Could you check a few things on this model? Use its own coordinates, in mm. A direction names the side the tool comes from. Coordinates: 2 decimals unless noted, no trailing zeros. One line per question, with ' | ' between items. Start each with the question number.
(1) I'm going to push flat-ended pins straight in: pin 1 Ø2.5 at (x, y) = (-150.5, 0.5) entering from -Z; pin 2 Ø10 at (x, z) = (-102, 42.5) entering from +Y; pin 3 Ø3 at (y, z) = (-116, -54) entering from +X. Where does each tip first touch, or does it pass through?
(2) If we mould it in two halves opening along X, with no side actions, what happens to faces 1 (the face through (-24, -8, 132.5)), 2 (the face through (-4, 1, 167.5)), 3 (the face through (-3.78, -130.33, -2.72))? For each: pulls with the +X half, pulls with the -X half, needs draft (parallel to the pull), parting line crosses it, or undercut.
(3) If I drill on line 1 along X through (y, z) = (24, 73.5); line 2 along X through (y, z) = (131, -10.5); line 3 along Y through (x, z) = (-90.5, 97.5), over which ranges is the centre line in solid material (lowest first)?
(4) Which directions (+Z, -Z, +X, -X, +Y, -Y) give clear straight access to the entire face, cutting with the end or side of a thin tool? Please do faces 4 (the face through (-4.336, 19.524, 119.856)), 5 (the face through (14, 161, -167.5)), 6 (the face through (-240.33, 2.24, -2.73)).
(5) Suppose I cut it at A-A (z = 68.5). Give the number of separate pieces and of enclosed holes in the cut face, plus the area to 3 significant figures.
```python
from build123d import *

# Parameters (mm, degrees)
F3_W      = 560
F3_H      = 340
F2_W      = 440
F2_H      = 220
F5_T      = -10
F8_R      = 40
F9_DEPTH  = 25
F10_R     = 20
F11_DEPTH = 25
F15_R     = 5
F6_R      = 2.5
F16_DEPTH = 75
F7_R      = 2.5
F17_DEPTH = 75


with BuildPart() as f4:
    # F3 (on offset) → F4 section 0
    with BuildSketch(Plane.XY.offset(-167.5)):
        Rectangle(F3_W, F3_H)
    # F2 (on offset) → F4 section 1
    with BuildSketch(Plane.XY.offset(167.5)):
        Rectangle(F2_W, F2_H)
    loft()

    # F5
    f5_openings = [f4.faces().sort_by_distance(p)[0] for p in [
        (0, 0, -167.5),
    ]]
    offset(amount=F5_T, openings=f5_openings)

    # F8 (on face) → F9 (join)
    with BuildSketch(Plane(origin=(0, 0, 157.5), x_dir=(1, 0, 0), z_dir=(0, 0, -1))):
        Circle(F8_R)
    extrude(amount=F9_DEPTH)

    # F10 (on face) → F11 (join)
    with BuildSketch(Plane(origin=(0, 0, 132.5), x_dir=(1, 0, 0), z_dir=(0, 0, -1))):
        Circle(F10_R)
    extrude(amount=F11_DEPTH)

    # F13 (on face) → F14 (revolve)
    with BuildSketch(Plane.XZ):
        with BuildLine():
            Line((0, 117.5), (0, 57.5))
            ThreePointArc((0, 57.5), (30, 87.5), (0, 117.5))
        make_face()
    revolve(axis=Axis((0, 0, 87.5), (0, 0, -1)))

    # F15
    f15_edges = [f4.edges().sort_by_distance(p)[0] for p in [
        (-20, 0, 132.5),
        (-40, 0, 132.5),
        (-20, 0, 109.86068),
        (-40, 0, 157.5),
    ]]
    fillet(f15_edges, radius=F15_R)

    # F6 (on face) → F16 (join, symmetric)
    with BuildSketch(Plane.XY.offset(167.5)):
        with Locations((-150, 0)):
            Circle(F6_R)
    extrude(amount=F16_DEPTH, both=True)

    # F7 (on face) → F17 (join, symmetric)
    with BuildSketch(Plane(origin=(242.2296568098, 0, 43.384416145), x_dir=(0, 1, 0), z_dir=(0.9843366432, 0, 0.1762991003))):
        with Locations((0, -89.2401358232)):
            Circle(F7_R)
    extrude(amount=F17_DEPTH, both=True)


solid = f4.part
```
Checks:
1) pin 1: stops at z = 92.5 | pin 2: stops at y = 133.28 | pin 3: stops at x = 259.94
2) face 1: undercut | face 2: needs draft | face 3: undercut
3) line 1: x = -236.84 to -226.68, -11.31 to 11.31, 226.68 to 236.84 | line 2: x = -251.88 to -241.72, 241.72 to 251.88 | line 3: y = -122.54 to -112.38, 112.38 to 122.54
4) face 4: none | face 5: -Z, +X, -X, +Y, -Y | face 6: -Z
5) separate pieces: 2 | enclosed holes: 1 | area: 16,100 mm^2
